Verification items for the finished model (mm, model axes). A direction names the side the tool comes from. Coordinates: 2 decimals unless noted, no trailing zeros. Write each loop counter-clockwise with the first axis right and the second up, starting at its lowest first coordinate (ties: lowest second). Pieces come first, ordered by that corner, then holes. Notation, with made-up numbers: (43, 47) -> (87, 47) arc R13 cw to (87, 52) -> close; hole circle Ø5 at (82.5, 73). An arc over 180 degrees is marked (long way). Answer in a Markdown table with one row per item.
```python
from build123d import *

# Parameters (mm, degrees)
SKETCH_1_R           = 1.5
EXTRUDE_1_DEPTH      = 4
SKETCH_2_R           = 3
CUT_EXTRUDE_1_DEPTH  = 3
SKETCH_3_W           = 32
SKETCH_3_H           = 44
EXTRUDE_2_DEPTH      = 40
SKETCH_4_R           = 1.5
CUT_EXTRUDE_2_DEPTH  = 65
SKETCH_5_R           = 3
CUT_EXTRUDE_10_DEPTH = 15
SKETCH_7_W           = 32
SKETCH_7_H           = 29.5
CUT_EXTRUDE_12_DEPTH = 28
CUT_EXTRUDE_11_DEPTH = 63


with BuildPart() as part:
    # 草图1 → 凸台-拉伸1 (new body)
    with BuildSketch(Plane.XY):
        with BuildLine():
            Line((-40, 32), (41, 32))
            ThreePointArc((41, 32), (43.828427125, 30.828427125), (45, 28))
            Line((45, 28), (45, 20))
            ThreePointArc((45, 20), (43.535533906, 16.464466094), (40, 15))
            Line((40, 15), (20, 15))
            ThreePointArc((20, 15), (16.464466094, 13.535533906), (15, 10))
            Line((15, 10), (15, -10))
            ThreePointArc((15, -10), (16.464466094, -13.535533906), (20, -15))
            Line((20, -15), (40, -15))
            ThreePointArc((40, -15), (43.535533906, -16.464466094), (45, -20))
            Line((45, -20), (45, -27))
            ThreePointArc((45, -27), (43.535533906, -30.535533906), (40, -32))
            Line((40, -32), (-40, -32))
            ThreePointArc((-40, -32), (-43.535533906, -30.535533906), (-45, -27))
            Line((-45, -27), (-45, 27))
            ThreePointArc((-45, 27), (-43.535533906, 30.535533906), (-40, 32))
        make_face()
        with Locations((-39.5, 23)):
            Circle(SKETCH_1_R, mode=Mode.SUBTRACT)
        with Locations((-39.5, -23)):
            Circle(SKETCH_1_R, mode=Mode.SUBTRACT)
        with Locations((39.5, -23)):
            Circle(SKETCH_1_R, mode=Mode.SUBTRACT)
        with Locations((39.5, 23)):
            Circle(SKETCH_1_R, mode=Mode.SUBTRACT)
    extrude(amount=EXTRUDE_1_DEPTH)

    # 草图2 → 切除-拉伸1 (cut)
    with BuildSketch(Plane.XY.offset(4)):
        with Locations((-39.5, 23)):
            Circle(SKETCH_2_R)
        with Locations((-39.5, -23)):
            Circle(SKETCH_2_R)
        with Locations((39.5, -23)):
            Circle(SKETCH_2_R)
        with Locations((39.5, 23)):
            Circle(SKETCH_2_R)
    extrude(amount=-CUT_EXTRUDE_1_DEPTH, mode=Mode.SUBTRACT)

    # 草图3 → 凸台-拉伸2 (add)
    with BuildSketch(Plane.XY.offset(4)):
        with Locations((-1, 10)):
            Rectangle(SKETCH_3_W, SKETCH_3_H)
    extrude(amount=EXTRUDE_2_DEPTH)

    # 草图4 → 切除-拉伸2 (cut, through all)
    with BuildSketch(Plane(origin=(0, 32, 0), x_dir=(1, 0, 0), z_dir=(0, 1, 0))):
        with Locations((-13, -13)):
            Circle(SKETCH_4_R)
        with Locations((-13, -33)):
            Circle(SKETCH_4_R)
        with Locations((10.7, -23)):
            Circle(SKETCH_4_R)
    extrude(amount=-CUT_EXTRUDE_2_DEPTH, mode=Mode.SUBTRACT)

    # 草图5 → 切除-拉伸10 (cut)
    with BuildSketch(Plane.XZ.offset(12)):
        with Locations((-13, 33)):
            Circle(SKETCH_5_R)
        with Locations((-13, 13)):
            Circle(SKETCH_5_R)
        with Locations((10.7, 23)):
            Circle(SKETCH_5_R)
    extrude(amount=-CUT_EXTRUDE_10_DEPTH, mode=Mode.SUBTRACT)

    # 草图7 → 切除-拉伸12 (cut)
    with BuildSketch(Plane(origin=(0, 32, 0), x_dir=(1, 0, 0), z_dir=(0, 1, 0))):
        with Locations((-1, -23)):
            Rectangle(SKETCH_7_W, SKETCH_7_H)
    extrude(amount=-CUT_EXTRUDE_12_DEPTH, mode=Mode.SUBTRACT)

    # 草图6 → 切除-拉伸11 (cut, through all)
    with BuildSketch(Plane.ZY.offset(17)):
        with BuildLine():
            Line((4, -12), (41.149391542, -0.855182537))
            ThreePointArc((41.149391542, -0.855182537), (43.209171713, 0.588400485), (44, 2.976122604))
            Line((44, 2.976122604), (44, -12))
            Line((44, -12), (4, -12))
        make_face()
        with BuildLine():
            Line((40, 32), (44, 32))
            Line((44, 32), (44, 28))
            ThreePointArc((44, 28), (42.828427125, 30.828427125), (40, 32))
        make_face()
    extrude(amount=-CUT_EXTRUDE_11_DEPTH, mode=Mode.SUBTRACT)


solid = part.part
```
1. Access from +Z, -Z, +X, -X, +Y, -Y to the whole of each face (thin tool, end or side, straight path). Record for faces 1 (the face through (-1, 18, 8.25)), 2 (the face through (44, 17, 2)), 3 (the face through (38, 22, 1)).
Findings below:
| item | result |
|---|---|
| face 1 | +X, -X, +Y |
| face 2 | +Z, -Z, +X |
| face 3 | +Z |
2. Sectioned sample at D-D, the plane y = -23. Record the cut outline in (x, z).
Findings below:
| item | result |
|---|---|
| outline | (-45, 0) -> (-41, 0) -> (-41, 1) -> (-42.5, 1) -> (-42.5, 4) -> (-45, 4) -> close; (-38, 0) -> (38, 0) -> (38, 1) -> (36.5, 1) -> (36.5, 4) -> (-36.5, 4) -> (-36.5, 1) -> (-38, 1) -> close; (41, 0) -> (45, 0) -> (45, 4) -> (42.5, 4) -> (42.5, 1) -> (41, 1) -> close |
3. Sectioned sample at A-A, the plane y = 23. Record the cut outline in (x, z).
Findings below:
| item | result |
|---|---|
| outline | (-45, 0) -> (-41, 0) -> (-41, 1) -> (-42.5, 1) -> (-42.5, 4) -> (-45, 4) -> close; (-38, 0) -> (38, 0) -> (38, 1) -> (36.5, 1) -> (36.5, 4) -> (15, 4) -> (15, 8.25) -> (-17, 8.25) -> (-17, 4) -> (-36.5, 4) -> (-36.5, 1) -> (-38, 1) -> close; (-17, 37.75) -> (15, 37.75) -> (15, 44) -> (-17, 44) -> close; (41, 0) -> (45, 0) -> (45, 4) -> (42.5, 4) -> (42.5, 1) -> (41, 1) -> close |
4. Sectioned sample at C-C, the plane x = -2. Record the cut outline in (y, z).
Findings below:
| item | result |
|---|---|
| outline | (-32, 0) -> (32, 0) -> (32, 8.25) -> (4, 8.25) -> (4, 37.75) -> (32, 37.75) -> (32, 40) arc R4 ccw to (28, 44) -> (2.98, 44) arc R4 ccw to (-0.86, 41.15) -> (-12, 4) -> (-32, 4) -> close |
5. Material ranges on probe 1 along Z at (x, y) = (-13, 3.8); probe 2 along Z at (x, y) = (7.5, 24); probe 3 along X at (y, z) = (-6, 13), recorded low to high. Write a range as from..to.
Findings below:
| item | result |
|---|---|
| probe 1 | z = 0..11.5, 14.5..31.5, 34.5..44 |
| probe 2 | z = 0..8.25, 37.75..44 |
| probe 3 | x = -17..-16, -10..15 |
6. Go/stop test with flat-tipped pins: pin 1 (3.5 mm diameter, centred on x = -13, z = 33, fed in from -Y); pin 2 (8 mm diameter, centred on x = -39.5, y = -23, fed in from +Z); pin 3 (5 mm diameter, centred on y = 21, z = 37.5, fed in from -X); pin 4 (2.5 mm diameter, centred on x = 10.7, z = 23, fed in from -Y). Record where each tip stops, or that it passes through.
Findings below:
| item | result |
|---|---|
| pin 1 | stops at y = 3 |
| pin 2 | stops at z = 4 |
| pin 3 | stops at x = -17 |
| pin 4 | passes through |
7. Release check for a two-part mould opening along Y. For faces 4 (the face through (10.505, 3.507, 21.513)), 5 (the face through (-1, 32, 39)), 6 (the face through (38.39, -21.99, 0.49)) record: released by +Y, released by -Y, zero draft, split by the parting line, or undercut.
Findings below:
| item | result |
|---|---|
| face 4 | zero draft |
| face 5 | released by +Y |
| face 6 | undercut |
8. Sectioned sample at B-B, the plane z = 23. Record the cut outline in (x, y), and give its area (3 significant figures).
Findings below:
| item | result |
|---|---|
| outline | (-17, -6.3) -> (7.7, -6.3) -> (7.7, 3) -> (9.2, 3) -> (9.2, 4) -> (-17, 4) -> close; (12.2, 3) -> (13.7, 3) -> (13.7, -6.3) -> (15, -6.3) -> (15, 4) -> (12.2, 4) -> close |
| area | 271 mm² |
